from build123d import *

# Parameters (mm, degrees)
SKETCH136_R   = 5.85
PAD069_DEPTH  = 2
SKETCH095_R   = 5.85
SKETCH095_R_2 = 3.75
PAD070_DEPTH  = 15
SKETCH096_R   = 8.5
PAD071_DEPTH  = 10


with BuildPart() as part:
    # Sketch136 → Pad069 (new body)
    with BuildSketch(Plane.XY):
        with Locations((-1.1, 0.5)):
            Circle(SKETCH136_R)
        Polygon((-4.408918, 5.231215), (-6.851811, 0), (-3.542893, -4.731215), (2.208918, -4.231215), (4.651811, 1), (1.342893, 5.731215), align=None, mode=Mode.SUBTRACT)
    extrude(amount=PAD069_DEPTH)

    # Sketch095 (on Face9 of Pad069) → Pad070 (join)
    with BuildSketch(Plane.XY.offset(2)):
        with Locations((-1.1, 0.5)):
            Circle(SKETCH095_R)
        with Locations((-1.1, 0.5)):
            Circle(SKETCH095_R_2, mode=Mode.SUBTRACT)
    extrude(amount=PAD070_DEPTH)

    # Sketch096 (on Face10 of Pad070) → Pad071 (join)
    with BuildSketch(Plane.XY.offset(17)):
        with Locations((-1.1, 0.5)):
            Circle(SKETCH096_R)
    extrude(amount=PAD071_DEPTH)


with BuildPart() as part_1:
    # Body010 placement: moved
    add(part.part.moved(Location((-5, -0.5, 43))))


solid = part_1.part
Geometry check sheet. Reference: the model listing, model coordinates, mm. A direction names the side the tool comes from. Give positions to 0.01 mm unless a question says otherwise; leave off trailing zeros. Write each loop counter-clockwise with the first axis right and the second up, starting at its lowest first coordinate (ties: lowest second). Pieces come first, ordered by that corner, then holes.
1) Go/stop test with flat-tipped pins: pin 1 Ø5 at (x, y) = (-5, -1.5) entering from -Z; pin 2 Ø3 at (y, z) = (6.5, 66) entering from +X; pin 3 Ø1 at (x, y) = (-12, -4) entering from -Z. Record where each tip stops, or that it passes through.
Values follow:
pin 1: stops at z = 45
pin 2: stops at x = 0.77
pin 3: stops at z = 60
2) Thickness scan on line 1 (Y direction, x = -6.1, z = 56.25); line 2 (Z direction, x = -10.25, y = 5.25); line 3 (X direction, y = -2.5, z = 48). Record the ranges inside material, lowest first.
Values follow:
line 1: y = -5.85 to -3.75, 3.75 to 5.85
line 2: z = 60 to 70
line 3: x = -11.39 to -8.9, -3.3 to -0.81
3) Cross-section at D-D (z = 65.75). Record the boundary of the cut face in (x, y), plus the area to 3 significant figures.
Values follow:
outline: circle Ø17 at (-6.1, 0)
area: 227 mm2
4) Cross-section at B-B (y = -3.25). Record the boundary of the cut face in (x, z).
Values follow:
outline: (-13.95, 60) - (-10.96, 60) - (-10.96, 43) - (-9.93, 43) - (-9.93, 45) - (-7.97, 45) - (-7.97, 60) - (-4.23, 60) - (-4.23, 45) - (-2.1, 45) - (-2.1, 43) - (-1.24, 43) - (-1.24, 60) - (1.75, 60) - (1.75, 70) - (-13.95, 70) - close
5) Set-up check for faces 1 (the face through (-14.59, 0.37, 64.93)), 2 (the face through (-8, -6, 60)): record each of +Z, -Z, +X, -X, +Y, -Y from which the full face is reachable in a straight line by a thin tool's end or side.
Values follow:
face 1: +Z, -Z
face 2: -Z
6) Release check for a two-part mould opening along X. For faces 3 (the face through (-0.696, -2.241, 51.381)), 4 (the face through (-6.1, 5.2, 43)), 5 (the face through (-1.98, 2.83, 43.99)) record: released by +X, released by -X, zero draft, split by the parting line, or undercut.
Values follow:
face 3: split by the parting line
face 4: zero draft
face 5: undercut
7) Cross-section at A-A (z = 47.5). Record the boundary of the cut face in (x, y).
Values follow:
outline: circle Ø11.7 at (-6.1, 0); hole circle Ø7.5 at (-6.1, 0)
8) Cross-section at C-C (x = -6.1). Record the boundary of the cut face in (y, z).
Values follow:
outline: (-8.5, 60) - (-5.85, 60) - (-5.85, 43) - (-5.02, 43) - (-5.02, 45) - (-3.75, 45) - (-3.75, 60) - (3.75, 60) - (3.75, 45) - (5.02, 45) - (5.02, 43) - (5.85, 43) - (5.85, 60) - (8.5, 60) - (8.5, 70) - (-8.5, 70) - close
